Model file for the job. Use its own axes, mm. A direction names the side the tool comes from. Give positions to 0.01 mm unless a question says otherwise; leave off trailing zeros. Loops run counter-clockwise (first coordinate to the right, second up) from the corner with the lowest first, then second, coordinate; pieces in that order, holes last. Notation, with made-up numbers: (-31, 51) - (-19, 51) arc R8 ccw to (-19, 65) - close; hole circle Ø3 at (-25, 33). An arc over 180 degrees is marked (long way). Use a Markdown table: item, result.
from build123d import *

# Parameters (mm, degrees)
FILLET1_R                = 0.1
SKETCH3_W                = 0.48
SKETCH3_H                = 2.1
SKETCH4_W                = 0.48
SKETCH4_H                = 0.68402847
RECPAT_COUNT             = 2
RECPAT_ANGLE             = 90
THDSCHPAT_COUNT          = 11
THDSCHPAT_PITCH          = 0.4
ESBO_O1_R                = 2.4
RESSALTO_EXTRUS_O1_DEPTH = 0.5


with BuildPart() as part:
    # BodySke → Base-Revolve (revolve)
    with BuildSketch(Plane.XY):
        with BuildLine():
            Line((1.6, 1), (1.6, 2))
            Line((1.6, 2), (1.1, 2))
            ThreePointArc((1.1, 2), (0.688403396, 1.885994341), (0.394117647, 1.576470588))
            ThreePointArc((0.394117647, 1.576470588), (0.100022625, 0.812494344), (0, 0))
            Line((0, 0), (20.6, 0))
            Line((20.6, 0), (20.6, 1))
            Line((20.6, 1), (1.6, 1))
        make_face()
    revolve(axis=Axis((-25.4, 0, 0), (1, 0, 0)))

    # Fillet1
    fillet1_edges = [part.edges().sort_by_distance(p)[0] for p in [
        (1.6, -1, 0),
    ]]
    fillet(fillet1_edges, radius=FILLET1_R)

    # Sketch3 → Recess section 0
    with BuildSketch(Plane(origin=(0, 0, 0), x_dir=(0, 0, -1), z_dir=(1, 0, 0))):
        Rectangle(SKETCH3_W, SKETCH3_H)
    # Sketch4 → Recess section 1
    with BuildSketch(Plane(origin=(1.42, 0, 0), x_dir=(0, 0, -1), z_dir=(1, 0, 0))):
        Rectangle(SKETCH4_W, SKETCH4_H)
    recess = loft(mode=Mode.SUBTRACT)

    # RecPat: Recess ×2 about axis
    recpat_axis = Axis((0, 0, 0), (1, 0, 0))
    for i in range(1, RECPAT_COUNT):
        add(recess.rotate(recpat_axis, i * RECPAT_ANGLE / (RECPAT_COUNT - 1)), mode=Mode.SUBTRACT)

    # RecCorSke → RecessCore (revolve, cut)
    with BuildSketch(Plane.XY):
        Polygon((0, 0), (0, 0.454796073), (1.42, 0.3555), (1.535508952, 0), align=None)
    revolve(axis=Axis((-3.175, 0, 0), (1, 0, 0)), mode=Mode.SUBTRACT)

    # ThdSchSke → ThreadSchematic (revolve, cut)
    with BuildSketch(Plane.XY):
        Polygon((16.6, -0.774), (16.441753096, -1), (16.441753096, -1.25), (16.758246904, -1.25), (16.758246904, -1), align=None)
    threadschematic = revolve(axis=Axis((-3.175, 0, 0), (1, 0, 0)), mode=Mode.SUBTRACT)

    # ThdSchPat: ThreadSchematic ×11
    with Locations(*[(i * THDSCHPAT_PITCH, 0, 0) for i in range(1, THDSCHPAT_COUNT)]):
        add(threadschematic, mode=Mode.SUBTRACT)

    # Esboço1 → Ressalto-extrusão1 (add)
    with BuildSketch(Plane(origin=(1.6, 0, 0), x_dir=(0, 0, -1), z_dir=(1, 0, 0))):
        Circle(ESBO_O1_R)
    extrude(amount=-RESSALTO_EXTRUS_O1_DEPTH)


solid = part.part
(1) Slice it at A-A, the plane x = 7. Write the cut outline in (y, z), plus the area to 3 significant figures.
Computed:
| item | result |
|---|---|
| outline | circle Ø2 at (0, 0) |
| area | 3.14 mm² |
(2) Pin check, flat tips, straight feed: P1, Ø2, axis at x = 10.5, z = -1.5, coming from the -Y side; P2, Ø2, axis at x = 6.5, y = 0.5, coming from the -Z side; P3, Ø1.5, axis at x = 14.5, z = 1, coming from the -Y side. Stop position of each tip, or through.
Computed:
| item | result |
|---|---|
| P1 | y = -0.87 |
| P2 | z = -1 |
| P3 | y = -0.97 |
(3) 3-axis set-ups, long thin cutter, end or side, ignore diameter. For faces 1 (the flat face through (1.1, 2, 1)), 2 (the cylindrical face through (1.354, 2.024, -1.29)): which of +Z, -Z, +X, -X, +Y, -Y reach the whole face in a straight line?
Computed:
| item | result |
|---|---|
| face 1 | -X |
| face 2 | +X, -X |
(4) Drill centre lines: probe 1 along Y at (x, z) = (8, 0.25); probe 2 along Z at (x, y) = (3, -0.85); probe 3 along X at (y, z) = (-2.1, -0.15). Where is each one in solid material? Low to high. Write a range as [from, to].
Computed:
| item | result |
|---|---|
| probe 1 | [-0.97, 0.97] |
| probe 2 | [-0.53, 0.53] |
| probe 3 | [1.1, 1.6] |
